from build123d import *

# Parameters (mm, degrees)
EXTRUDE1_DEPTH = 75
EXTRUDE2_DEPTH = 70
EXTRUDE3_DEPTH = 10
SKETCH6_R      = 207.5
EXTRUDE4_DEPTH = 0.01


with BuildPart() as part:
    # Sketch1 → Extrude1 (new body, symmetric)
    with BuildSketch(Plane.XY):
        Polygon((0, 0), (0, 30), (60, 64.641016151), (60, 0), align=None)
    extrude(amount=EXTRUDE1_DEPTH, both=True)

    # Sketch2 → Extrude2 (add)
    with BuildSketch(Plane(origin=(0, 0, 0), x_dir=(1, 0, 0), z_dir=(0, 1, 0))):
        Polygon((0, 37.141798985), (-33.301270189, 10.224702754), (-33.301270189, -10.224702754), (0, -37.141798985), align=None)
    extrude(amount=EXTRUDE2_DEPTH)

    # Sketch3 → Extrude3 (add)
    with BuildSketch(Plane(origin=(0, 70, 0), x_dir=(-1, 0, 0), z_dir=(0, 1, 0))):
        Polygon((0, -50), (43.301270189, -15), (43.301270189, 15), (0, 50), align=None)
    extrude(amount=EXTRUDE3_DEPTH)

    # Sketch4 → Loft1 section 0
    with BuildSketch(Plane(origin=(0, 80, 0), x_dir=(-1, 0, 0), z_dir=(0, 1, 0)), mode=Mode.PRIVATE) as loft1_s0:
        Polygon((0, -50), (43.301270189, -15), (43.301270189, 15), (0, 50), align=None)
    loft([loft1_s0.sketch, Vertex(0, 105, 0)])

    # Sketch6 → Extrude4 (add)
    with BuildSketch(Plane(origin=(0, 0, 0), x_dir=(1, 0, 0), z_dir=(0, 1, 0))):
        with Locations(Location((8.349364905, 0.109485549, 0), (0, 0, 270))):  # turned: the seam where the file's is
            Circle(SKETCH6_R)
    extrude(amount=EXTRUDE4_DEPTH)


solid = part.part
Model file for the job. Use its own axes, mm. A direction names the side the tool comes from. Coordinates: 2 decimals unless noted, no trailing zeros. Write each loop counter-clockwise with the first axis right and the second up, starting at its lowest first coordinate (ties: lowest second). Pieces come first, ordered by that corner, then holes. Notation, with made-up numbers: (68.25, 46.5) -> (103.25, 46.5) arc R21 cw to (103.25, 73.5) -> close; hole circle Ø4 at (-18.75, 23.25). An arc over 180 degrees is marked (long way). One line per item, written item: value. Start each with the question number.
1) Slice it at A-A on y = 13. Write the cut outline in (x, z).
2) Flat gauge pins, fed straight in: pin 1 Ø8 at (y, z) = (63.5, -21) entering from -X; pin 2 Ø2 at (x, z) = (-83, 124.5) entering from +Y; pin 3 Ø11 at (y, z) = (73.5, -6) entering from -X. Where does each tip first touch, or does it go through?
3) Pull direction Y, two halves, no side cores. Call faces 4 (the face through (37, 26, -75)), 5 (the face through (-34, 70, -7)), 6 (the face through (-14.39, 87.12, -24.13)): +Y half, -Y half, draft (parallel to the pull), parting line (faces both ways), or undercut.
4) Which spindle directions (+Z, -Z, +X, -X, +Y, -Y) get a long thin tool onto all of the face, cutting with end or side? Do faces 1 (the face through (29.58, 47.08, 1.05)), 2 (the face through (-16.884, 34.515, 23.495)), 3 (the face through (37, 26, 75)). Say none if no direction does.
5) Probe probe 1 along X at (y, z) = (43, -12.5); probe 2 along Z at (x, y) = (50, 20.5); probe 3 along Z at (x, y) = (-11.5, 45.5). List the from-to ranges inside material, lowest first.
6) Slice it at B-B on y = 54. Write the cut outline in (x, z).
Answers follow:
1. outline: (-33.3, -10.22) -> (0, -37.14) -> (0, -75) -> (60, -75) -> (60, 75) -> (0, 75) -> (0, 37.14) -> (-33.3, 10.22) -> close
2. pin 1: x = -24.92
2. pin 2: y = 0.01
2. pin 3: x = -43.3
3. face 4: draft
3. face 5: undercut
3. face 6: +Y half
4. face 1: +Z, -Z, +Y
4. face 2: +Z, -X
4. face 3: +Z, +X, -X, +Y
5. probe 1: -30.49 to 0, 22.52 to 60
5. probe 2: -75 to 75
5. probe 3: -27.85 to 27.85
6. outline: (-33.3, -10.22) -> (0, -37.14) -> (0, 37.14) -> (-33.3, 10.22) -> close; (41.57, -75) -> (60, -75) -> (60, 75) -> (41.57, 75) -> close
